Build history of the part. All positions in model axes, mm. A direction names the side the tool comes from. Round coordinates to 2 decimals unless told otherwise and drop trailing zeros. Order: outer loops, then holes, each group sorted by start corner. A loop starts at its lowest first (then second) coordinate and runs counter-clockwise, first axis right, second up. Notation, with made-up numbers: M 22,75.25 L 56,75.25 A17 ccw 56,100.25 Z; hole C 18,83 d1. An arc over 180 degrees is marked long. Use CSV: the item, a comma, the result in double quotes.
from build123d import *

# Parameters (mm, degrees)
SKETCH1_R           = 31.75
BASE_EXTRUDE_DEPTH  = 14.2875
SKETCH2_R           = 15.113
BOSS_EXTRUDE1_DEPTH = 38.1
SKETCH3_R           = 6.35
CUT_EXTRUDE1_DEPTH  = 77.724
SKETCH5_R           = 2.54
CUT_EXTRUDE3_DEPTH  = 37.846
SKETCH6_R           = 4.1275
CUT_EXTRUDE4_DEPTH  = 25.8572
SKETCH7_R           = 4.1275
CUT_EXTRUDE5_DEPTH  = 15.24
SKETCH8_R           = 4.1275
CUT_EXTRUDE6_DEPTH  = 26.51
SKETCH9_R           = 4.1275
CUT_EXTRUDE7_DEPTH  = 10.508
CHAMFER1_SIZE       = 0.508


with BuildPart() as part:
    # Sketch1 → Base-Extrude (new body)
    with BuildSketch(Plane.XY):
        Circle(SKETCH1_R)
    extrude(amount=BASE_EXTRUDE_DEPTH)

    # Sketch2 → Boss-Extrude1 (add)
    with BuildSketch(Plane.XY):
        with Locations(Location((0, 0, 0), (0, 0, 180))):
            Circle(SKETCH2_R)
    extrude(amount=BOSS_EXTRUDE1_DEPTH)

    # Sketch3 → Cut-Extrude1 (cut)
    with BuildSketch(Plane.XY):
        with Locations(Location((0, 0, 0), (0, 0, 180))):
            Circle(SKETCH3_R)
    extrude(amount=CUT_EXTRUDE1_DEPTH, mode=Mode.SUBTRACT)

    # Sketch5 → Cut-Extrude3 (cut)
    with BuildSketch(Plane(origin=(38.336621827, 0, 0), x_dir=(0, 0, -1), z_dir=(1, 0, 0))):
        with Locations((-31.75, 0)):
            Circle(SKETCH5_R)
    extrude(amount=-CUT_EXTRUDE3_DEPTH, mode=Mode.SUBTRACT)

    # Sketch6 → Cut-Extrude4 (cut)
    with BuildSketch(Plane(origin=(38.336621827, 0, 0), x_dir=(0, 0, -1), z_dir=(1, 0, 0))):
        with Locations((-7.14375, 0)):
            Circle(SKETCH6_R)
    cut_extrude4 = extrude(amount=-CUT_EXTRUDE4_DEPTH, mode=Mode.SUBTRACT)

    # Sketch7 → Cut-Extrude5 (cut)
    with BuildSketch(Plane(origin=(0, 27.700210809, 0), x_dir=(-1, 0, 0), z_dir=(0, 1, 0))):
        with Locations(Location((0, 7.14375, 0), (0, 0, 90))):
            Circle(SKETCH7_R)
    cut_extrude5 = extrude(amount=-CUT_EXTRUDE5_DEPTH, mode=Mode.SUBTRACT)

    # Mirror1: Cut-Extrude4 across plane
    add(cut_extrude4.mirror(Plane(origin=(0, 0, 0), x_dir=(0, 0, 1), z_dir=(1, 0, 0))), mode=Mode.SUBTRACT)

    # Mirror2: Cut-Extrude5 across plane
    add(cut_extrude5.mirror(Plane.ZX), mode=Mode.SUBTRACT)

    # Sketch8 → Cut-Extrude6 (cut)
    with BuildSketch(Plane(origin=(0, 27.700210809, 0), x_dir=(-1, 0, 0), z_dir=(0, 1, 0))):
        with Locations(Location((0, 7.14375, 0), (0, 0, 90))):
            Circle(SKETCH8_R)
    extrude(amount=CUT_EXTRUDE6_DEPTH, mode=Mode.SUBTRACT)

    # Sketch9 → Cut-Extrude7 (cut)
    with BuildSketch(Plane(origin=(0, -34.128089617, 0), x_dir=(-1, 0, 0), z_dir=(0, 1, 0))):
        with Locations(Location((0, 7.14375, 0), (0, 0, 270))):
            Circle(SKETCH9_R)
    extrude(amount=CUT_EXTRUDE7_DEPTH, mode=Mode.SUBTRACT)

    # Chamfer1
    chamfer1_edges = [part.edges().sort_by_distance(p)[0] for p in [
        (6.35, 0, 0),
        (-31.75, 0, 0),
        (-31.75, 0, 14.2875),
        (15.113, 0, 38.1),
    ]]
    chamfer(chamfer1_edges, length=CHAMFER1_SIZE)


solid = part.part
(1) Drop flat-ended pins along their axis: pin 1 (1 mm diameter, centred on x = 0, y = -16, fed in from +Z); pin 2 (1 mm diameter, centred on x = -9, z = 9, fed in from +Y); pin 3 (2.5 mm diameter, centred on x = 1.5, z = 9, fed in from +Y). Give the stop position or say it passes through.
Answer block:
pin 1,"stops at z = 14.29"
pin 2,"stops at y = 30.59"
pin 3,"stops at y = 12.46"
(2) Wall check: line 1 (Z direction, x = 0, y = 22); line 2 (Y direction, x = 0, z = 30); line 3 (Y direction, x = 0, z = 8). Give the ranges that are in metal, low to high. Write a range as from..to.
Answer block:
line 1,"z = 0..3.02, 11.27..14.29"
line 2,"y = -15.11..-6.35, 6.35..15.11"
line 3,"y = -12.46..-6.35, 6.35..12.46"
(3) Two-plate mould, pull along Z, no slides. Class faces 6 (the face through (0.4, -7.4, 0)), 7 (the face through (-6, 3, 38.1)), 8 (the face through (22.25, 0.181, 11.267)): released by +Z, released by -Z, zero draft, split by the parting line, or undercut.
Answer block:
face 6,"released by -Z"
face 7,"released by +Z"
face 8,"undercut"
(4) Cut at C-C, the plane z = 36. Give the cut face in (x, y).
Answer block:
outline,"C 0,0 d30.23; hole C 0,0 d12.7"
(5) Cut at D-D, the plane z = 2. Give the cut face in (x, y), and give its area (3 significant figures).
Answer block:
outline,"C 0,0 d63.5; hole C 0,0 d12.7"
area,"3,040 mm²"
(6) Tool access for faces 1 (the face through (0.18, 21.97, 3.02)), 2 (the face through (-22.251, 0.181, 11.267)), 3 (the face through (-14.415, -4.54, 25.777)), 4 (the face through (0, -12.46, 7)), 5 (the face through (10.531, 0.112, 34.288)): list every direction of +Z, -Z, +X, -X, +Y, -Y with a clear straight run to the whole face (end or side of a thin tool).
Answer block:
face 1,"+Y"
face 2,"-X"
face 3,"+Z"
face 4,"-Y"
face 5,"+X"
(7) Cut at B-B, the plane y = 0. Count the separate pieces of the cut face and the enclosed holes in it, and give its area (3 significant figures).
Answer block:
separate pieces,"3"
enclosed holes,"0"
area,"779 mm²"
